Model file for the job. Use its own axes, mm. A direction names the side the tool comes from. Give positions to 0.01 mm unless a question says otherwise; leave off trailing zeros. Loops run counter-clockwise (first coordinate to the right, second up) from the corner with the lowest first, then second, coordinate; pieces in that order, holes last. Notation, with made-up numbers: (-5, 36) - (5, 36) arc R25 cw to (5, 58) - close; hole circle Ø9 at (60, 70). An arc over 180 degrees is marked (long way). Use a Markdown table: item, result.
from build123d import *

# Parameters (mm, degrees)
SKETCH1_R         = 40
WHEEL_BLANK_DEPTH = 1.5
T_SLOT_DEPTH      = 2.5
CIRPATTERN_COUNT  = 12
SKETCH3_R         = 4
CENTER_HOLE_DEPTH = 6
CIRPATTERN1_COUNT = 6


with BuildPart() as part:
    # Sketch1 → Wheel Blank (new body)
    with BuildSketch(Plane(origin=(0, 0, 0), x_dir=(1, 0, 0), z_dir=(0, 1, 0))):
        Circle(SKETCH1_R)
    extrude(amount=WHEEL_BLANK_DEPTH)

    # Sketch2 → T-Slot (cut, through all)
    with BuildSketch(Plane(origin=(0, 0, 0), x_dir=(1, 0, 0), z_dir=(0, 1, 0))):
        with BuildLine():
            Line((-1.395979868, 39.975633081), (-1.343630623, 38.47654684))
            ThreePointArc((-1.343630623, 38.47654684), (-3.188115989, 38.367771846), (-5.0252584, 38.170627163))
            ThreePointArc((-5.0252584, 38.170627163), (-5.88617707, 37.048656109), (-4.764206016, 36.18773744))
            ThreePointArc((-4.764206016, 36.18773744), (0, 36.5), (4.764206016, 36.18773744))
            ThreePointArc((4.764206016, 36.18773744), (5.88617707, 37.048656109), (5.0252584, 38.170627163))
            ThreePointArc((5.0252584, 38.170627163), (3.188115989, 38.367771846), (1.343630623, 38.47654684))
            Line((1.343630623, 38.47654684), (1.395979868, 39.975633081))
            ThreePointArc((1.395979868, 39.975633081), (0, 40), (-1.395979868, 39.975633081))
        make_face()
    t_slot = extrude(amount=T_SLOT_DEPTH, mode=Mode.SUBTRACT)

    # CirPattern: T-Slot ×12 about axis
    cirpattern_axis = Axis((0, 0, 0), (0, 1, 0))
    for i in range(1, CIRPATTERN_COUNT):
        add(t_slot.rotate(cirpattern_axis, i * 360 / CIRPATTERN_COUNT), mode=Mode.SUBTRACT)

    # Sketch3 → Center Hole (cut)
    with BuildSketch(Plane(origin=(0, 0, 0), x_dir=(1, 0, 0), z_dir=(0, 1, 0))):
        Circle(SKETCH3_R)
    extrude(amount=CENTER_HOLE_DEPTH, mode=Mode.SUBTRACT)

    # Sketch4 → M3 Clearance Hole1 (revolve, cut)
    with BuildSketch(Plane(origin=(2.610523844, 1.5, -19.828897227), x_dir=(0, 0, 1), z_dir=(1, 0, 0))):
        Polygon((0, 0), (0, 10.751075774), (1.25, 10), (1.25, 0), align=None)
    m3_clearance_hole1 = revolve(axis=Axis((2.610523844, 7.85, -19.828897227), (0, -1, 0)), mode=Mode.SUBTRACT)

    # CirPattern1: M3 Clearance Hole1 ×6 about axis
    cirpattern1_axis = Axis((0, 0, 0), (0, 1, 0))
    for i in range(1, CIRPATTERN1_COUNT):
        add(m3_clearance_hole1.rotate(cirpattern1_axis, i * 360 / CIRPATTERN1_COUNT), mode=Mode.SUBTRACT)


solid = part.part
(1) Pin check, flat tip, straight feed: P1, Ø2, axis at x = -18.48, z = 7.65, coming from the -Y side. Stop position of the tip, or through.
Computed:
| item | result |
|---|---|
| P1 | through |
(2) Slice it at A-A, the plane z = 0. Write the cut outline in (x, y), plus the area to 3 significant figures.
Computed:
| item | result |
|---|---|
| outline | (-36.5, 0) - (-4, 0) - (-4, 1.5) - (-36.5, 1.5) - close; (4, 0) - (36.5, 0) - (36.5, 1.5) - (4, 1.5) - close |
| area | 97.5 mm² |
(3) 3-axis set-ups, long thin cutter, end or side, ignore diameter. For faces 1 (the cylindrical face through (-18.308, 0.74, -31.576)), 2 (the cylindrical face through (38.67, 0.74, -10.23)): which of +Z, -Z, +X, -X, +Y, -Y reach the whole face in a straight line?
Computed:
| item | result |
|---|---|
| face 1 | +Y, -Y |
| face 2 | -Z, +X, +Y, -Y |
(4) Slice it at C-C, the plane x = 10.5. Write the cut outline in (y, z), plus the area to 3 significant figures.
Computed:
| item | result |
|---|---|
| outline | (0, -38.6) - (1.5, -38.6) - (1.5, 38.6) - (0, 38.6) - close |
| area | 116 mm² |
(5) Drill centre lines: probe 1 along X at (y, z) = (0.55, 16); probe 2 along Z at (x, y) = (-32, 0.5); probe 3 along X at (y, z) = (0.8, -15). Where is each one in solid material? Low to high. Write a range as [from, to].
Computed:
| item | result |
|---|---|
| probe 1 | [-36.66, -35.02], [-32.81, 32.81], [35.02, 36.66] |
| probe 2 | [-24, -21.41], [-17.56, 17.56], [21.41, 24] |
| probe 3 | [-37.08, -35.46], [-33.28, 33.28], [35.46, 37.08] |
(6) Slice it at B-B, the plane x = 0. Write the cut outline in (y, z), plus the area to 3 significant figures.
Computed:
| item | result |
|---|---|
| outline | (0, -36.5) - (1.5, -36.5) - (1.5, -4) - (0, -4) - close; (0, 4) - (1.5, 4) - (1.5, 36.5) - (0, 36.5) - close |
| area | 97.5 mm² |
(7) Mould opens along Z. For faces 3 (the cylindrical face through (-10.23, 0.74, -38.67)), 4 (the flat face through (8, 1.5, -1)), 5 (the cylindrical face through (31.643, 0.74, 18.192)) say: pulls with the +Z half, pulls with the -Z half, needs draft (parallel to the pull), parting line crosses it, or undercut.
Computed:
| item | result |
|---|---|
| face 3 | pulls with the -Z half |
| face 4 | needs draft |
| face 5 | undercut |
(8) Slice it at D-D, the plane y = 0.9. Count the separate pieces of the cut face and the enclosed holes in it, plus the area to 3 significant figures.
Computed:
| item | result |
|---|---|
| separate pieces | 1 |
| enclosed holes | 7 |
| area | 4,620 mm² |
